Could you check a few things on this model? Use its own coordinates, in mm. A direction names the side the tool comes from. Give positions to 0.01 mm unless a question says otherwise; leave off trailing zeros. Write each loop counter-clockwise with the first axis right and the second up, starting at its lowest first coordinate (ties: lowest second). Pieces come first, ordered by that corner, then holes. Notation, with made-up numbers: M 1.5,-7.75 L 5.5,-7.75 A16 ccw 5.5,19.25 Z; hole C 16,39.5 d3. An arc over 180 degrees is marked long. Answer as CSV lines item,"result". Start each with the question number.
from build123d import *

# Parameters (mm, degrees)
EXTRU_MINCE1_DEPTH           = 13.5
ENL_V_MAT_EXTRU_1_DEPTH      = 3.45
ENL_V_MAT_EXTRU_1_DEPTH_BACK = 4.001688959


with BuildPart() as part:
    # Esquisse1 → Extru.-Mince1 (new body, symmetric)
    with BuildSketch(Plane.XY):
        Polygon((-24, -0.95), (-21.016167821, 2.45), (-10.50808391, -2.45), (0, 2.45), (10.50808391, -2.45), (21.016167821, 2.45), (24, -0.95), (23.624195852, -1.279804855), (20.887672756, 1.838392808), (10.50808391, -3.001688959), (0, 1.898311041), (-10.50808391, -3.001688959), (-20.887672756, 1.838392808), (-23.624195852, -1.279804855), align=None)
    extrude(amount=EXTRU_MINCE1_DEPTH, both=True)

    # Esquisse2 → Enlèv. mat.-Extru.1 (cut, two sides)
    with BuildSketch(Plane(origin=(0, 0, 0), x_dir=(1, 0, 0), z_dir=(0, 1, 0))) as enl_v_mat_extru_1_sk:
        with BuildLine():
            Line((-12.5, 7.5), (12.5, 7.5))
            ThreePointArc((12.5, 7.5), (20, 0), (12.5, -7.5))
            Line((12.5, -7.5), (-12.5, -7.5))
            ThreePointArc((-12.5, -7.5), (-20, 0), (-12.5, 7.5))
        make_face()
    extrude(amount=ENL_V_MAT_EXTRU_1_DEPTH, mode=Mode.SUBTRACT)
    extrude(enl_v_mat_extru_1_sk.sketch, amount=-ENL_V_MAT_EXTRU_1_DEPTH_BACK, mode=Mode.SUBTRACT)


solid = part.part
1. On a 3-axis mill with a long thin cutter (end or side, diameter ignored), from which of +Z, -Z, +X, -X, +Y, -Y can I reach the whole of each face in a straight line? I mean faces 1 (the flat face through (-20.238, 1.536, 0.189)), 2 (the flat face through (20.359, 2.143, 0.189)), 3 (the cylindrical face through (-20, 1.8, 0.1)), 4 (the flat face through (22.49, 0.77, 0.19)). Say none if no direction works.
2. Imagine slicing it at A-A, the plane z = 0. Please give me the cut outline in (x, y).
3. Please list where these lines run through material, in increasing order: line 1 (X direction, y = 1.5, z = -12.5); line 2 (X direction, y = 0.05, z = 7.25); line 3 (X direction, y = -1.15, z = -12).
4. Imagine slicing it at C-C, the plane z = 8. Please give me the cut outline in (x, y), plus the area to 3 significant figures.
5. Will these pins go through, and if not, where does the flat tip stop? P1, Ø10, axis at x = -4, z = 8, coming from the -Y side; P2, Ø1.6, axis at x = -3.5, y = -1, coming from the -Z side; P3, Ø1.5, axis at y = 0.5, z = 5.5, coming from the +X side; P4, Ø3, axis at x = 17, z = 5.5, coming from the +Y side.
6. Thinking about a two-plate mould opening in X: for faces 5 (the flat face through (-22.529, 0.726, 0.189)), 6 (the flat face through (5.328, -0.586, -10.458)), 7 (the flat face through (-1.7, 1.4, 13.5)), which applies, pulls with the +X half, pulls with the -X half, needs draft (parallel to the pull), parting line crosses it, or undercut?
7. Imagine slicing it at B-B, the plane x = -8.5. Please give me the cut outline in (y, z), plus the area to 3 significant figures.
Solutions:
1,face 1,"+Z, -Z, -Y"
1,face 2,"+Z, -Z, +Y"
1,face 3,"+Y, -Y"
1,face 4,"+Z, -Z, +X, +Y"
2,outline,"M -24,-0.95 L -23.62,-1.28 L -20.89,1.84 L -20,1.42 L -20,1.98 L -21.02,2.45 Z; M 20,1.42 L 20.89,1.84 L 23.62,-1.28 L 24,-0.95 L 21.02,2.45 L 20,1.98 Z"
3,line 1,"-21.85 to -21.18, -20.16 to -18.98, -2.04 to -0.85, 0.85 to 2.04, 18.98 to 20.16, 21.18 to 21.85"
3,line 2,"-23.12 to -22.46, -17.05 to -15.87, 15.87 to 17.05, 22.46 to 23.12"
3,line 3,"-23.77 to -23.51, -14.48 to -13.3, -7.72 to -6.54, 6.54 to 7.72, 13.3 to 14.48, 23.51 to 23.77"
4,outline,"M -24,-0.95 L -23.62,-1.28 L -20.89,1.84 L -10.51,-3 L 0,1.9 L 10.51,-3 L 20.89,1.84 L 23.62,-1.28 L 24,-0.95 L 21.02,2.45 L 10.51,-2.45 L 0,2.45 L -10.51,-2.45 L -21.02,2.45 Z"
4,area,"27.5 mm²"
5,P1,"y = -2.3"
5,P2,"through"
5,P3,"x = 23.39"
5,P4,"y = 1.28"
6,face 5,"pulls with the -X half"
6,face 6,"undercut"
6,face 7,"needs draft"
7,outline,"M -2.07,-13.5 L -1.51,-13.5 L -1.51,-7.5 L -2.07,-7.5 Z; M -2.07,7.5 L -1.51,7.5 L -1.51,13.5 L -2.07,13.5 Z"
7,area,"6.62 mm²"
